from build123d import *

# Parameters (mm, degrees)
SKETCH2_R          = 4.7625
BASE_EXTRUDE_DEPTH = 12.7
BASE_EXTRUDE_TAPER = 3
FILLET1_R          = 3.175
SKETCH3_R          = 3.175
CUT_EXTRUDE1_DEPTH = 6.35


with BuildPart() as part:
    # Sketch2 → Base-Extrude (new body)
    with BuildSketch(Plane(origin=(0, 0, 0), x_dir=(1, 0, 0), z_dir=(0, 1, 0))):
        Circle(SKETCH2_R)
    extrude(amount=BASE_EXTRUDE_DEPTH, taper=BASE_EXTRUDE_TAPER)

    # Fillet1
    fillet1_edges = [part.edges().sort_by_distance(p)[0] for p in [
        (-4.7625, 0, 0),
    ]]
    fillet(fillet1_edges, radius=FILLET1_R)

    # Sketch3 → Cut-Extrude1 (cut)
    with BuildSketch(Plane(origin=(0, 12.7, 0), x_dir=(-1, 0, 0), z_dir=(0, 1, 0))):
        with Locations(Location((0, 0, 0), (0, 0, 90))):
            Circle(SKETCH3_R)
    extrude(amount=-CUT_EXTRUDE1_DEPTH, mode=Mode.SUBTRACT)


solid = part.part
Build history of the part. All positions in model axes, mm. A direction names the side the tool comes from. Round coordinates to 2 decimals unless told otherwise and drop trailing zeros. Write each loop counter-clockwise with the first axis right and the second up, starting at its lowest first coordinate (ties: lowest second). Pieces come first, ordered by that corner, then holes. Notation, with made-up numbers: M -32,53.25 L -6,53.25 A15 cw -6,68.25 Z; hole C -35.5,15.5 d8. An arc over 180 degrees is marked long. Use CSV: the item, a comma, the result in double quotes.
1. Wall check: probe 1 along Y at (x, z) = (-1, -1); probe 2 along Z at (x, y) = (-2, 8.25); probe 3 along Z at (x, y) = (-0.75, 12) (3 decimals). Give the ranges that are in metal, low to high. Write a range as from..to.
Reply:
probe 1,"y = 0..6.35"
probe 2,"z = -3.84..-2.47, 2.47..3.84"
probe 3,"z = -4.065..-3.085, 3.085..4.065"
2. Saw through at A-A (y = 7.25). Give the cut face in (x, z) (3 decimals), plus the area to 3 significant figures.
Reply:
outline,"C 0,0 d8.765; hole C 0,0 d6.35"
area,"28.7 mm²"
3. Flat gauge pins, fed straight in: pin 1 (3 mm diameter, centred on y = 10, z = -1.5, fed in from -X); pin 2 (1.5 mm diameter, centred on x = -0.5, y = 7, fed in from +Z); pin 3 (3 mm diameter, centred on x = -0.5, y = 5.5, fed in from +Z). Where does each tip first touch, or does it go through?
Reply:
pin 1,"stops at x = -4.28"
pin 2,"stops at z = 4.43"
pin 3,"stops at z = 4.55"
4. Saw through at C-C (y = 8.75). Give the cut face in (x, z) (3 decimals).
Reply:
outline,"C 0,0 d8.608; hole C 0,0 d6.35"
5. Saw through at B-B (y = 3.75). Give the cut face in (x, z), plus the area to 3 significant figures.
Reply:
outline,"C 0,0 d9.13"
area,"65.5 mm²"
6. Tool access for faces 4 (the face through (2, 12.7, 3)), 5 (the face through (-1.93, 9.57, -2.52)): list every direction of +Z, -Z, +X, -X, +Y, -Y with a clear straight run to the whole face (end or side of a thin tool).
Reply:
face 4,"+Z, -Z, +X, -X, +Y"
face 5,"+Y"
7. Two-plate mould, pull along X, no slides. Class faces 1 (the face through (0, 6.35, 0)), 2 (the face through (4.14, 8.09, -1.3)), 3 (the face through (0, 0, 0)): +X half, -X half, draft (parallel to the pull), parting line (faces both ways), or undercut.
Reply:
face 1,"undercut"
face 2,"parting line"
face 3,"draft"
